For this review, take the finished solid that the model builds, in its own axes (mm). Coordinates: 2 decimals unless noted, no trailing zeros. Loops run counter-clockwise (first coordinate to the right, second up) from the corner with the lowest first, then second, coordinate; pieces in that order, holes last. Notation, with made-up numbers: M -31,-15.75 L 28,-15.75 A26 ccw 28,14.25 Z; hole C 15.25,-33 d3. An arc over 180 degrees is marked long. Use one line per item in the form item = value.
Autodesk Fusion 360 part; units mm, degrees
sketch "Sketch1" plane through (0, 0, 0) normal (0, 0, 1) x (1, 0, 0)
  line L0 (0, 0) -> (-230, 0)
  line L1 (-230, 0) -> (-230, 120)
  line L2 (-230, 120) -> (0, 120)
  line L3 (0, 120) -> (0, 0)
  dimension "d1" = 120
  dimension "d2" = 230
extrude "Extrude1" add sketch "Sketch1" along normal blind 80
sketch "Sketch2" plane through (0, 0, 80) normal (0, 0, 1) x (-1, 0, 0)
  line L0 (0, -120) -> (230, -120)
  line L1 (230, -120) -> (230, 0)
  line L2 (230, 0) -> (0, 0)
  line L3 (0, 0) -> (0, -120)
  circle A0 centre (115, -120) radius 107.5
  dimension "d5" = 215
extrude "Extrude2" cut sketch "Sketch2" against normal blind 170 contours L0 A0 picked at (128.0914, -86.6437)
fillet "Fillet1" radius 2 10 edges at (-222.5, 120, 40) (-230, 120, 40) (-7.5, 120, 40) (0, 120, 40) (-115, 12.5, 80) (-115, 12.5, 0) (-3.75, 120, 80) (-3.75, 120, 0) (-226.25, 120, 80) (-226.25, 120, 0)
1. Draft analysis for pull direction X (two halves, no side actions). For faces 1 (the face through (-230, 58, 39)), 2 (the face through (-133, 11, 0)), 3 (the face through (-117.336, 12.525, 40.532)), state which applies: +X half, -X half, draft (parallel to the pull), parting line (faces both ways), or undercut.
Computed values:
face_1 = -X half
face_2 = draft
face_3 = undercut
2. Consider section B-B on x = -115. Write out the cut boundary in (y, z), plus the area to 3 significant figures.
Computed values:
outline = M 0,0 L 10.5,0 A2 ccw 12.5,2 L 12.5,78 A2 ccw 10.5,80 L 0,80 Z
area = 998 mm2
3. Wall thickness on line 1 along X through (y, z) = (32, 39); line 2 along X through (y, z) = (55.5, 59); line 3 along Y through (x, z) = (-164.5, 53): over which ranges is each line inside the solid? List them lowest first. Write a range as from..to.
Computed values:
line_1 = -230..-176.74, -53.26..0
line_2 = -230..-201, -29..0
line_3 = 0..24.57
4. Consider section A-A on z = 46. Write out the cut boundary in (x, y).
Computed values:
outline = M -230,0 L 0,0 L 0,118 A2 ccw -2,120 L -5.52,120 A2 ccw -7.52,118.04 A107.5 cw -222.48,118.04 A2 ccw -224.48,120 L -228,120 A2 ccw -230,118 Z
5. For pin 1 Ø5 at (x, z) = (-26, 56) entering from +Y; pin 2 Ø6 at (x, z) = (-123.5, 57.5) entering from +Y; pin 3 Ø4 at (x, z) = (-189, 22) entering from -Y; pin 4 Ø3 at (x, z) = (-47.5, 60.5) entering from +Y, all flat-tipped, find the tip position at first contact; note any pin that passes through.
Computed values:
pin_1 = 63.57
pin_2 = 13.12
pin_3 = 0
pin_4 = 37.57
